The listing builds one solid part. Answer for the finished solid, in the listing's coordinates (mm). A direction names the side the tool comes from. Round coordinates to 2 decimals unless told otherwise and drop trailing zeros. Order: outer loops, then holes, each group sorted by start corner. A loop starts at its lowest first (then second) coordinate and runs counter-clockwise, first axis right, second up. Notation, with made-up numbers: (33.5, 50) - (43.5, 50) arc R12 ccw to (43.5, 67) - close; hole circle Ø7 at (57, 0). An arc over 180 degrees is marked (long way). One line per item, written item: value. Start each with the question number.
1. Section A-A, the plane y = 0.5 is taken. Give the vertices of the cut face in (x, z).
2. A flat-ended cylindrical pin translates along its axis: P1, Ø0.5, axis at y = 1, z = 0.5, coming from the -X side. Find the tip coordinate at first contact, or state that the pin passes through.
3. A tool of negligible diameter and unlimited length cuts with its end or side. For faces 5 (the flat face through (-2.6, 0.8, 0.4)), 6 (the flat face through (0, -3, 0)), from which of +Z, -Z, +X, -X, +Y, -Y can it reach the whole face along a straight path? Write none if from no direction.
4. Straight lines are drawn through the part: line 1 (X direction, y = 0, z = 0.5); line 2 (X direction, y = -1.25, z = 0.8); line 3 (Y direction, x = 1.75, z = 0.1). For each, find the intervals that lie inside material, in ascending order.
5. For a pull along X with two mould halves and no side action, classify faces 1 (the flat face through (0, -3, 1)), 2 (the flat face through (2.6, 0.8, 0.4)), 3 (the cylindrical face through (-0.138, -4.938, 0.493)), 4 (the cylindrical face through (-0.1, -2.6, 0.5)) as released by +X, released by -X, zero draft, split by the parting line, or undercut.
6. Section C-C, the plane y = 1.75 is taken. Give the vertices of the cut face in (x, z), then the cut area to 3 significant figures.
7. Section B-B, the plane x = 3.5 is taken. Give the vertices of the cut face in (y, z) (3 decimals), then the cut area to 3 significant figures.
8. Section D-D, the plane z = 0.6 is taken. Give the vertices of the cut face in (x, y).
from build123d import *

# Parameters (mm, degrees)
PAD001_DEPTH = 5
PAD_DEPTH    = 1
FILLET_R     = 1


with BuildPart() as pad001:
    # Sketch001 → Pad001 (new body, symmetric)
    with BuildSketch(Plane.YZ):
        Polygon((0, 1), (3, 0), (3, 1), align=None)
    extrude(amount=PAD001_DEPTH, both=True)


with BuildPart() as fillet_body:
    # Sketch → Pad (new body)
    with BuildSketch(Plane.XY):
        with BuildLine():
            ThreePointArc((-4.513812, 2.006138), (4e-06, -4.939543), (4.513808, 2.006146))
            ThreePointArc((4.513808, 2.006146), (3.392408, 2.578216), (2.6, 1.600007))
            Line((2.6, 1.600007), (2.6, 0))
            ThreePointArc((-2.6, 0), (0, -2.6), (2.6, 0))
            Line((-2.6, 1.599999), (-2.6, 0))
            ThreePointArc((-2.6, 1.599999), (-3.392408, 2.578216), (-4.513812, 2.006138))
        make_face()
    extrude(amount=PAD_DEPTH)

    # Cut: cut Pad001
    add(pad001.part, mode=Mode.SUBTRACT)

    # Fillet
    fillet_edges = [fillet_body.edges().sort_by_distance(p)[0] for p in [
        (3.769772, 0, 1),
        (-3.769772, 0, 1),
    ]]
    fillet(fillet_edges, radius=FILLET_R)


solid = fillet_body.part
Answer list:
1. outline: (-4.91, 0) - (-2.6, 0) - (-2.6, 0.83) - (-4.91, 0.83) - close; (2.6, 0) - (4.91, 0) - (4.91, 0.83) - (2.6, 0.83) - close
2. P1: stops at x = -4.88
3. face 5: +Z, -Z, +Y
3. face 6: -Z, +X, -X, +Y, -Y
4. line 1: x = -4.94 to -2.6, 2.6 to 4.94
4. line 2: x = -4.78 to -2.28, 2.28 to 4.78
4. line 3: y = -4.62 to -1.92
5. face 1: zero draft
5. face 2: undercut
5. face 3: split by the parting line
5. face 4: undercut
6. outline: (-4.62, 0) - (-2.61, 0) - (-2.61, 0.42) - (-4.62, 0.42) - close; (2.61, 0) - (4.62, 0) - (4.62, 0.42) - (2.61, 0.42) - close
6. area: 1.67 mm²
7. outline: (-3.486, 0) - (2.595, 0) - (2.595, 0.135) - (0.154, 0.949) arc R1 ccw to (-0.162, 1) - (-3.486, 1) - close
7. area: 4.96 mm²
8. outline: (-4.79, 1.2) arc R4.94 ccw (long way) to (4.79, 1.2) - (2.6, 1.2) - (2.6, 0) arc R2.6 cw to (-2.6, 0) - (-2.6, 1.2) - close
